Design review of the part built by this model. Coordinates are the model's own, in mm. Face numbers are marked on the shaded views. Coordinates: 2 decimals unless noted, no trailing zeros. Loops run counter-clockwise (first coordinate to the right, second up) from the corner with the lowest first, then second, coordinate; pieces in that order, holes last. Notation, with made-up numbers: (61, -4.75) -> (104, -4.75) arc R12 ccw to (104, 3.25) -> close; hole circle Ø8 at (86, 70). An arc over 180 degrees is marked (long way). Use a Markdown table: item, result. Add a question column.
Q1. For probe 1 along X at (y, z) = (8.5, 0.45); probe 2 along X at (y, z) = (24.5, 2.15); probe 3 along Y at (x, z) = (-32.5, 1.8), list the stretches that pass through material, from the lowest coordinate up.
Q2. Take a section at A-A on x = -29.5. Write out the cut boundary in (y, z), plus the area to 3 significant figures.
Q3. Draft analysis for pull direction Y (two halves, no side actions). For the marked faces 1 and 2, state which applies: pulls with the +Y half, pulls with the -Y half, needs draft (parallel to the pull), parting line crosses it, or undercut.
Q4. Take a section at B-B on y = 11. Write out the cut boundary in (x, z).
Q5. Take a section at D-D on x = -33. Write out the cut boundary in (y, z), plus the area to 3 significant figures.
Q6. Clearance check with flat-ended pins moving along their axes: pin 1 Ø5.5 at (x, y) = (-24.74, 14.67) entering from +Z; pin 2 Ø1.2 at (x, z) = (-19.5, 1) entering from +Y. State where each tip first meets the part, or that it passes through.
Q7. Take a section at C-C on z = 0.6. Write out the cut boundary in (x, y), plus the area to 3 significant figures.
from build123d import *

# Parameters (mm, degrees)
F0_W     = 6.5
F0_H     = 4.75
F0_R     = 1.5
F0_R_2   = 3
F1_DEPTH = 2.5


with BuildPart() as f1:
    # F0 (on Top) → F1 (new body)
    with BuildSketch(Plane.XY):
        Polygon((-39.987817, 27.423815), (-39.987817, 1.923815), (-9.487817, 1.923815), (-9.487817, 27.423815), (-15.487817, 27.423815), (-15.487817, 21.423815), (-21.987817, 21.423815), (-21.987817, 27.423815), align=None)
        with Locations((-31.737817, 9.298815)):
            Rectangle(F0_W, F0_H, mode=Mode.SUBTRACT)
        with Locations((-24.737817, 8.548815)):
            Circle(F0_R, mode=Mode.SUBTRACT)
        with Locations((-32.562817, 14.673815)):
            Circle(F0_R, mode=Mode.SUBTRACT)
        with Locations((-24.737817, 14.673815)):
            Circle(F0_R_2, mode=Mode.SUBTRACT)
        with Locations((-24.737817, 20.798815)):
            Circle(F0_R, mode=Mode.SUBTRACT)
        with Locations((-16.912817, 14.673815)):
            Circle(F0_R, mode=Mode.SUBTRACT)
    extrude(amount=F1_DEPTH)


solid = f1.part
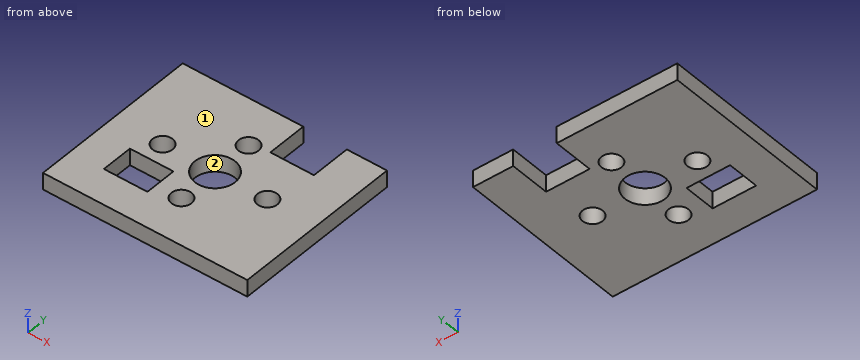
Answer list:
| question | item | result |
|---|---|---|
| 1 | probe 1 | -39.99 to -34.99, -28.49 to -26.24, -23.24 to -9.49 |
| 1 | probe 2 | -39.99 to -21.99, -15.49 to -9.49 |
| 1 | probe 3 | 1.92 to 6.92, 11.67 to 13.18, 16.17 to 27.42 |
| 2 | outline | (1.92, 0) -> (6.92, 0) -> (6.92, 2.5) -> (1.92, 2.5) -> close; (11.67, 0) -> (27.42, 0) -> (27.42, 2.5) -> (11.67, 2.5) -> close |
| 2 | area | 51.9 mm² |
| 3 | face 1 | needs draft |
| 3 | face 2 | undercut |
| 4 | outline | (-39.99, 0) -> (-34.99, 0) -> (-34.99, 2.5) -> (-39.99, 2.5) -> close; (-28.49, 0) -> (-9.49, 0) -> (-9.49, 2.5) -> (-28.49, 2.5) -> close |
| 5 | outline | (1.92, 0) -> (6.92, 0) -> (6.92, 2.5) -> (1.92, 2.5) -> close; (11.67, 0) -> (13.24, 0) -> (13.24, 2.5) -> (11.67, 2.5) -> close; (16.11, 0) -> (27.42, 0) -> (27.42, 2.5) -> (16.11, 2.5) -> close |
| 5 | area | 44.7 mm² |
| 6 | pin 1 | through |
| 6 | pin 2 | y = 21.42 |
| 7 | outline | (-39.99, 1.92) -> (-9.49, 1.92) -> (-9.49, 27.42) -> (-15.49, 27.42) -> (-15.49, 21.42) -> (-21.99, 21.42) -> (-21.99, 27.42) -> (-39.99, 27.42) -> close; hole (-34.99, 6.92) -> (-28.49, 6.92) -> (-28.49, 11.67) -> (-34.99, 11.67) -> close; hole circle Ø3 at (-32.56, 14.67); hole circle Ø6 at (-24.74, 14.67); hole circle Ø3 at (-24.74, 8.55); hole circle Ø3 at (-24.74, 20.8); hole circle Ø3 at (-16.91, 14.67) |
| 7 | area | 651 mm² |
